The listing builds one solid part. Answer for the finished solid, in the listing's coordinates (mm). Face numbers are marked on the shaded views. Round coordinates to 2 decimals unless told otherwise and drop trailing zeros. Loops run counter-clockwise (first coordinate to the right, second up) from the corner with the lowest first, then second, coordinate; pieces in that order, holes last. Notation, with made-up numbers: (17.5, 60.25) -> (70.5, 60.25) arc R9 ccw to (70.5, 71.25) -> close; hole circle Ø4 at (36.5, 71). An arc over 180 degrees is marked (long way). Use a Markdown table: item, result. Add a question column.
Q1. For a pull along Y with two mould halves and no side action, classify the marked faces 1, 2, 3 and 4 as released by +Y, released by -Y, zero draft, split by the parting line, or undercut.
Q2. Section B-B on y = 17 is taken. Give the vertices of the cut face in (x, z) (3 decimals), then the cut area to 3 significant figures.
Q3. Section A-A on x = 5.75 is taken. Give the vertices of the cut face in (y, z), then the cut area to 3 significant figures.
Q4. Section C-C on z = 3 is taken. Give the vertices of the cut face in (x, y), then the cut area to 3 significant figures.
Q5. Section D-D on x = 8.25 is taken. Give the vertices of the cut face in (y, z).
Q6. Given pin 1 Ø3 at (x, z) = (14, 38.5) entering from -Y; pin 2 Ø10 at (y, z) = (4, 4.5) entering from -X; pin 3 Ø2 at (x, z) = (3.5, 35) entering from -Y, each flat-ended and moving along its own axis, determine where each tip first touches the part or whether it passes through.
Q7. Consider line 1 (X direction, y = 17, z = 23); line 2 (Y direction, x = 2.5, z = 35); line 3 (Y direction, x = 1, z = 33). Determine where each line is inside the solid, lowest interval first.
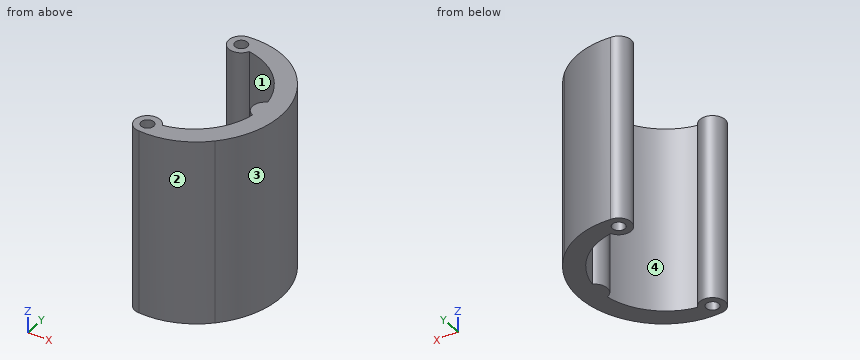
from build123d import *

# Parameters (mm, degrees)
BOSS_EXTRUDE1_DEPTH             = 44
F_3_0MM_DOWEL_HOLE1_D           = 3
F_3_0MM_DOWEL_HOLE1_CSINK_D     = 3.05
F_3_0MM_DOWEL_HOLE1_CSINK_ANGLE = 100


with BuildPart() as part:
    # Sketch1 → Boss-Extrude1 (new body)
    with BuildSketch(Plane(origin=(0, 0, 0), x_dir=(0, 1, 0), z_dir=(0, 0, 1))):
        with BuildLine():
            ThreePointArc((14.594339842, -14.594339842), (18.893257917, -7.888351803), (20, 0))
            ThreePointArc((20, 0), (15.373021566, 2.520504151), (15.764705882, -2.733870597))
            ThreePointArc((15.764705882, -2.733870597), (11.313708499, -11.313708499), (2.733870597, -15.764705882))
            ThreePointArc((2.733870597, -15.764705882), (0, -14), (-2.733870597, -15.764705882))
            ThreePointArc((-2.733870597, -15.764705882), (-11.313708499, -11.313708499), (-15.764705882, -2.733870597))
            ThreePointArc((-15.764705882, -2.733870597), (-15.373021566, 2.520504151), (-20, 0))
            ThreePointArc((-20, 0), (-18.893257917, -7.888351803), (-14.594339842, -14.594339842))
            ThreePointArc((-14.594339842, -14.594339842), (0, -20.639513339), (14.594339842, -14.594339842))
        make_face()
    extrude(amount=BOSS_EXTRUDE1_DEPTH)

    # Ø3.0mm Dowel Hole1 (through all)
    with Locations(Plane(origin=(0, 0, 0), x_dir=(1, 0, 0), z_dir=(0, 0, -1))):
        with Locations((0, -17), (0, 17)):
            CounterSinkHole(F_3_0MM_DOWEL_HOLE1_D / 2, F_3_0MM_DOWEL_HOLE1_CSINK_D / 2, counter_sink_angle=F_3_0MM_DOWEL_HOLE1_CSINK_ANGLE)


solid = part.part
Checked values:
| question | item | result |
|---|---|---|
| 1 | face 1 | undercut |
| 1 | face 2 | released by -Y |
| 1 | face 3 | split by the parting line |
| 1 | face 4 | undercut |
| 2 | outline | (-3, 0) -> (-1.525, 0) -> (-1.5, 0.021) -> (-1.5, 44) -> (-3, 44) -> close; (1.5, 0.021) -> (1.525, 0) -> (11.637, 0) -> (11.637, 44) -> (1.5, 44) -> close |
| 2 | area | 512 mm2 |
| 3 | outline | (-19.54, 0) -> (-14.93, 0) -> (-14.93, 44) -> (-19.54, 44) -> close; (14.93, 0) -> (19.54, 0) -> (19.54, 44) -> (14.93, 44) -> close |
| 3 | area | 406 mm2 |
| 4 | outline | (0, -20) arc R18.64 ccw to (14.59, -14.59) arc R20.64 ccw to (14.59, 14.59) arc R18.64 ccw to (0, 20) arc R3 ccw (long way) to (2.73, 15.76) arc R16 cw to (15.76, 2.73) arc R3 ccw to (15.76, -2.73) arc R16 cw to (2.73, -15.76) arc R3 ccw (long way) to start; hole circle Ø3 at (0, -17); hole circle Ø3 at (0, 17) |
| 4 | area | 290 mm2 |
| 5 | outline | (-18.76, 0) -> (-13.71, 0) -> (-13.71, 44) -> (-18.76, 44) -> close; (13.71, 0) -> (18.76, 0) -> (18.76, 44) -> (13.71, 44) -> close |
| 6 | pin 1 | stops at y = -16.4 |
| 6 | pin 2 | stops at x = 13.23 |
| 6 | pin 3 | stops at y = -20.02 |
| 7 | line 1 | x = -3 to -1.5, 1.5 to 11.64 |
| 7 | line 2 | y = -20.02 to -15.34, 15.34 to 20.02 |
| 7 | line 3 | y = -20.05 to -18.12, -15.88 to -14.17, 14.17 to 15.88, 18.12 to 20.05 |
